Input: part model. Units: mm. Frame: model coordinates. A direction names the side the tool comes from. Round coordinates to 2 decimals unless told otherwise and drop trailing zeros. Loops run counter-clockwise (first coordinate to the right, second up) from the corner with the lowest first, then second, coordinate; pieces in that order, holes last.
(1) Access query for faces 4 (the face through (-100.35, 6.549, 23.698)), 5 (the face through (-50.875, 6.958, -48.081)). Directions: +Z, -Z, +X, -X, +Y, -Y. A direction counts if a zero-diameter tool reaches every point of the face in a straight line with its end or side. Return the directions, or none.
(2) Draft query along Z for faces 1 (the face through (0, 5, -65)), 2 (the face through (-30.8, 5.3, 59.7)), 3 (the face through (-22, 5, -40)). Return one class per face: released by +Z, released by -Z, zero draft, split by the parting line, or undercut.
(3) Cut plane D-D, the plane x = 55. Output: boundary loops of the cut face in (y, z), and give its area (3 significant figures).
(4) Cut plane C-C, the plane x = -75. Output: boundary loops of the cut face in (y, z).
(5) First-contact query: pin 1 Ø8 at (x, z) = (45.5, 11.5) entering from -Y; pin 2 Ø4 at (x, z) = (-101, 19) entering from +Y; pin 3 Ø5.5 at (y, z) = (6.5, -54) entering from -X; pin 4 Ø3.5 at (x, z) = (15, 55) entering from -Y. Flat tips, straight axial feed; report the tip coordinate or a pass-through.
(6) Line query: line 1 (X direction, y = 6.25, z = 0); line 2 (Z direction, x = 19, y = 8.5); line 3 (X direction, y = 9.5, z = 24). Output: solid intervals per line, ascending.
(7) Cut plane B-B, the plane z = 35. Output: boundary loops of the cut face in (x, y).
(8) Cut plane A-A, the plane z = 0. Output: boundary loops of the cut face in (x, y).
from build123d import *

# Parameters (mm, degrees)
SKETCH1_R                = 70
BOSS_EXTRUDE1_DEPTH      = 10
CUT_EXTRUDE1_DEPTH       = 100.498743711
CUT_EXTRUDE1_DEPTH_BACK  = 100.498743711
CUT_EXTRUDE2_DEPTH       = 100.498743711
CUT_EXTRUDE2_DEPTH_BACK  = 100.498743711
SKETCH3_R                = 2.75
CUT_EXTRUDE3_START       = -10
CUT_EXTRUDE3_DEPTH       = 7
SKETCH5_W                = 80
SKETCH5_H                = 80
BOSS_EXTRUDE2_DEPTH      = 10
CHAMFER1_SIZE            = 4
CUT_EXTRUDE4_DEPTH       = 7
CUT_EXTRUDE5_DEPTH       = 142.215903639
CUT_EXTRUDE5_DEPTH_BACK  = 142.215903639
SKETCH7_R                = 2.75
CUT_EXTRUDE6_DEPTH       = 142.396362897
CUT_EXTRUDE6_DEPTH_BACK  = 142.396362897
CUT_EXTRUDE7_DEPTH       = 142.396362897
CUT_EXTRUDE7_DEPTH_BACK  = 142.396362897
CHAMFER3_SIZE            = 5
CUT_EXTRUDE8_DEPTH       = 142.396362897
CUT_EXTRUDE8_DEPTH_BACK  = 142.396362897
SKETCH10_R               = 2.75
SKETCH11_R               = 3.55
CUT_EXTRUDE9_DEPTH       = 9
CUT_EXTRUDE11_DEPTH      = 142.396362897
CUT_EXTRUDE11_DEPTH_BACK = 142.396362897
SKETCH12_OUTSIDE_W       = 242.084
SKETCH12_OUTSIDE_H       = 189.638


with BuildPart() as part:
    # Sketch1 → Boss-Extrude1 (new body)
    with BuildSketch(Plane(origin=(0, 0, 0), x_dir=(1, 0, 0), z_dir=(0, 1, 0))):
        with Locations(Location((0, 0, 0), (0, 0, 270))):
            Circle(SKETCH1_R)
    extrude(amount=BOSS_EXTRUDE1_DEPTH)

    # Sketch2 → Cut-Extrude1 (cut, two sides: drawn at the far end of the back side and taken through both)
    with BuildSketch(Plane(origin=(0, 10, 0), x_dir=(1, 0, 0), z_dir=(0, 1, 0)).offset(-CUT_EXTRUDE1_DEPTH_BACK)):
        with BuildLine():
            Line((0, -40), (-130.143973447, -40))
            ThreePointArc((-130.143973447, -40), (-170.143973447, 0), (-130.143973447, 40))
            Line((-130.143973447, 40), (0, 40))
            ThreePointArc((0, 40), (40, 0), (0, -40))
        make_face()
    extrude(amount=CUT_EXTRUDE1_DEPTH + CUT_EXTRUDE1_DEPTH_BACK, mode=Mode.SUBTRACT)

    # Sketch3 → Cut-Extrude2 (cut, two sides: drawn at the far end of the back side and taken through both)
    with BuildSketch(Plane(origin=(0, 0, 0), x_dir=(-1, 0, 0), z_dir=(0, -1, 0)).offset(-CUT_EXTRUDE2_DEPTH_BACK)):
        with Locations(Location((15, 55, 0), (0, 0, 90))):
            Circle(SKETCH3_R)
        with Locations(Location((-15, 55, 0), (0, 0, 90))):
            Circle(SKETCH3_R)
        with Locations(Location((-15, -55, 0), (0, 0, 270))):
            Circle(SKETCH3_R)
        with Locations(Location((15, -55, 0), (0, 0, 270))):
            Circle(SKETCH3_R)
    extrude(amount=CUT_EXTRUDE2_DEPTH + CUT_EXTRUDE2_DEPTH_BACK, mode=Mode.SUBTRACT)

    # Sketch4 → Cut-Extrude3 (cut)
    with BuildSketch(Plane.XZ.offset(CUT_EXTRUDE3_START)):
        Polygon((-15, -50.092522712), (-19.25, -52.546261356), (-19.25, -57.453738644), (-15, -59.907477288), (-10.75, -57.453738644), (-10.75, -52.546261356), align=None)
        Polygon((15, -50.092522712), (10.75, -52.546261356), (10.75, -57.453738644), (15, -59.907477288), (19.25, -57.453738644), (19.25, -52.546261356), align=None)
        Polygon((-15, 59.907477288), (-19.25, 57.453738644), (-19.25, 52.546261356), (-15, 50.092522712), (-10.75, 52.546261356), (-10.75, 57.453738644), align=None)
        Polygon((15, 59.907477288), (10.75, 57.453738644), (10.75, 52.546261356), (15, 50.092522712), (19.25, 52.546261356), (19.25, 57.453738644), align=None)
    extrude(amount=CUT_EXTRUDE3_DEPTH, mode=Mode.SUBTRACT)

    # Sketch5 → Boss-Extrude2 (add)
    with BuildSketch(Plane.XZ):
        with Locations((-82.445626465, 0)):
            Rectangle(SKETCH5_W, SKETCH5_H)
    extrude(amount=-BOSS_EXTRUDE2_DEPTH)

    # Chamfer1
    chamfer1_edges = [part.edges().sort_by_distance(p)[0] for p in [
        (70, 0, 0),
    ]]
    chamfer(chamfer1_edges, length=CHAMFER1_SIZE)

    # Sketch6 → Cut-Extrude4 (cut)
    with BuildSketch(Plane(origin=(0, 10, 0), x_dir=(1, 0, 0), z_dir=(0, 1, 0))):
        Polygon((-102.445626465, 24.907477288), (-106.695626465, 22.453738644), (-106.695626465, 17.546261356), (-102.445626465, 15.092522712), (-98.195626465, 17.546261356), (-98.195626465, 22.453738644), align=None)
        Polygon((-102.445626465, -15.092522712), (-106.695626465, -17.546261356), (-106.695626465, -22.453738644), (-102.445626465, -24.907477288), (-98.195626465, -22.453738644), (-98.195626465, -17.546261356), align=None)
    extrude(amount=-CUT_EXTRUDE4_DEPTH, mode=Mode.SUBTRACT)

    # Sketch7 → Cut-Extrude5 (cut, two sides: drawn at the far end of the back side and taken through both)
    with BuildSketch(Plane(origin=(0, 3, 0), x_dir=(1, 0, 0), z_dir=(0, 1, 0)).offset(-CUT_EXTRUDE5_DEPTH_BACK)):
        with Locations(Location((-102.402760328, 20, 0), (0, 0, 270))):
            Circle(SKETCH7_R)
        with Locations(Location((-102.402760328, -20, 0), (0, 0, 270))):
            Circle(SKETCH7_R)
    extrude(amount=CUT_EXTRUDE5_DEPTH + CUT_EXTRUDE5_DEPTH_BACK, mode=Mode.SUBTRACT)

    # Sketch8 → Cut-Extrude6 (cut, two sides: drawn at the far end of the back side and taken through both)
    with BuildSketch(Plane(origin=(0, 10, 0), x_dir=(1, 0, 0), z_dir=(0, 1, 0)).offset(-CUT_EXTRUDE6_DEPTH_BACK)):
        Polygon((-57.445626465, -40), (-132.928087077, -22.5), (-132.928087077, 22.5), (-57.445626465, 40), (-157.567703317, 66.574038668), (-157.567703317, -80.170037604), align=None)
    extrude(amount=CUT_EXTRUDE6_DEPTH + CUT_EXTRUDE6_DEPTH_BACK, mode=Mode.SUBTRACT)

    # Sketch9 → Cut-Extrude7 (cut, two sides: drawn at the far end of the back side and taken through both)
    with BuildSketch(Plane.XZ.offset(-CUT_EXTRUDE7_DEPTH_BACK)):
        with BuildLine():
            Line((-61.450221561, 30), (-42.445626465, 40))
            Line((-42.445626465, 40), (0, 30))
            ThreePointArc((0, 30), (30, 0), (0, -30))
            Line((0, -30), (-42.445626465, -40))
            Line((-42.445626465, -40), (-61.450221561, -30))
            ThreePointArc((-61.450221561, -30), (-91.450221561, 0), (-61.450221561, 30))
        make_face()
    extrude(amount=CUT_EXTRUDE7_DEPTH + CUT_EXTRUDE7_DEPTH_BACK, mode=Mode.SUBTRACT)

    # Chamfer3
    chamfer3_edges = [part.edges().sort_by_distance(p)[0] for p in [
        (-122.445626465, 0, 0),
    ]]
    chamfer(chamfer3_edges, length=CHAMFER3_SIZE)

    # Sketch10 → Cut-Extrude8 (cut, two sides: drawn at the far end of the back side and taken through both)
    with BuildSketch(Plane.XZ.offset(-CUT_EXTRUDE8_DEPTH_BACK)):
        with Locations(Location((55, 0, 0), (0, 0, 270))):
            Circle(SKETCH10_R)
    extrude(amount=CUT_EXTRUDE8_DEPTH + CUT_EXTRUDE8_DEPTH_BACK, mode=Mode.SUBTRACT)

    # Sketch11 → Cut-Extrude9 (cut)
    with BuildSketch(Plane(origin=(0, 10, 0), x_dir=(1, 0, 0), z_dir=(0, 1, 0))):
        with Locations(Location((55, 0, 0), (0, 0, 270))):
            Circle(SKETCH11_R)
    extrude(amount=-CUT_EXTRUDE9_DEPTH, mode=Mode.SUBTRACT)

    # Sketch12 outside → Cut-Extrude11 (cut, two sides: drawn at the far end of the back side and taken through both)
    with BuildSketch(Plane(origin=(0, 10, 0), x_dir=(1, 0, 0), z_dir=(0, 1, 0)).offset(-CUT_EXTRUDE11_DEPTH_BACK)):
        with Locations((-26.223, 0)):
            Rectangle(SKETCH12_OUTSIDE_W, SKETCH12_OUTSIDE_H)
        with BuildLine():
            Line((-122.445626465, 24.93027399), (-18.547305729, 64.349685667))
            ThreePointArc((-18.547305729, 64.349685667), (-16.803211487, 64.836077894), (-15, 65))
            Line((-15, 65), (15, 65))
            ThreePointArc((15, 65), (19.537776451, 63.91114947), (23.087360843, 60.881716977))
            Line((23.087360843, 60.881716977), (63.087360843, 5.881716977))
            ThreePointArc((63.087360843, 5.881716977), (65, 0), (63.087360843, -5.881716977))
            Line((63.087360843, -5.881716977), (23.087360843, -60.881716977))
            ThreePointArc((23.087360843, -60.881716977), (19.537776451, -63.91114947), (15, -65))
            Line((15, -65), (-15, -65))
            ThreePointArc((-15, -65), (-16.803211487, -64.836077894), (-18.547305729, -64.349685667))
            Line((-18.547305729, -64.349685667), (-122.445626465, -24.93027399))
            Line((-122.445626465, -24.93027399), (-122.445626465, 24.93027399))
        make_face(mode=Mode.SUBTRACT)
    extrude(amount=CUT_EXTRUDE11_DEPTH + CUT_EXTRUDE11_DEPTH_BACK, mode=Mode.SUBTRACT)


solid = part.part
Reported:
1. face 4: +Y
1. face 5: -Z, -X, +Y, -Y
2. face 1: released by -Z
2. face 2: released by +Z
2. face 3: undercut
3. outline: (0, -17) - (10, -17) - (10, -3.55) - (1, -3.55) - (1, -2.75) - (0, -2.75) - close; (0, 2.75) - (1, 2.75) - (1, 3.55) - (10, 3.55) - (10, 17) - (0, 17) - close
3. area: 271 mm2
4. outline: (0, -35.93) - (10, -35.93) - (10, -26.77) - (0, -26.77) - close; (0, 26.77) - (10, 26.77) - (10, 35.93) - (0, 35.93) - close
5. pin 1: stops at y = 0
5. pin 2: stops at y = 3
5. pin 3: stops at x = -47.68
5. pin 4: passes through
6. line 1: x = -122.45 to -91.45, 40 to 51.45, 58.55 to 65
6. line 2: z = -64.17 to -57.6, -52.4 to -35.2, 35.2 to 52.4, 57.6 to 64.17
6. line 3: x = -122.45 to -104.02, -100.87 to -79.45, 32 to 49.91
7. outline: (-79.01, 0) - (-51.95, 0) - (-51.95, 10) - (-79.01, 10) - close; (19.36, 0) - (41.91, 0) - (41.91, 10) - (19.36, 10) - close
8. outline: (-122.45, 5) - (-117.45, 0) - (-91.45, 0) - (-91.45, 10) - (-122.45, 10) - close; (40, 0) - (52.25, 0) - (52.25, 1) - (51.45, 1) - (51.45, 10) - (40, 10) - close; (57.75, 0) - (65, 0) - (65, 10) - (58.55, 10) - (58.55, 1) - (57.75, 1) - close
